Here's how the part is built. I have some questions about the finished solid (model axes, mm). Face numbers are marked on the shaded views. Give positions to 0.01 mm unless a question says otherwise; leave off trailing zeros. Loops run counter-clockwise (first coordinate to the right, second up) from the corner with the lowest first, then second, coordinate; pieces in that order, holes last. Notation, with made-up numbers: (-32.75, 53.5) - (14.25, 53.5) arc R23 ccw to (14.25, 66.5) - close; hole circle Ø7 at (40, 81). An arc over 180 degrees is marked (long way). Use a Markdown table: item, result.
from build123d import *

# Parameters (mm, degrees)
F0_R     = 1.1811
F0_R_2   = 1.5875
F1_DEPTH = 0.79375
F2_SIZE2 = 0.127
F2_SIZE  = 0.127


with BuildPart() as f1:
    # F0 (on Front) → F1 (new body, symmetric)
    with BuildSketch(Plane.XZ):
        with BuildLine():
            Line((5.280381, 3.991776), (-7.04344, 3.991776))
            ThreePointArc((-7.04344, 3.991776), (-3.637121, -4.925726), (5.280381, -1.519407))
            Line((5.280381, -1.519407), (5.280381, 3.991776))
        make_face()
        with Locations((-0.881529, -3.777536)):
            Circle(F0_R, mode=Mode.SUBTRACT)
        with Locations((-0.881529, 1.236185)):
            Circle(F0_R_2, mode=Mode.SUBTRACT)
    extrude(amount=F1_DEPTH, both=True)

    # F2
    f2_edges = [f1.edges().sort_by_distance(p)[0] for p in [
        (-2.062629, -0.79375, -3.777536),
    ]]
    chamfer(f2_edges, length=F2_SIZE, length2=F2_SIZE2)


solid = f1.part
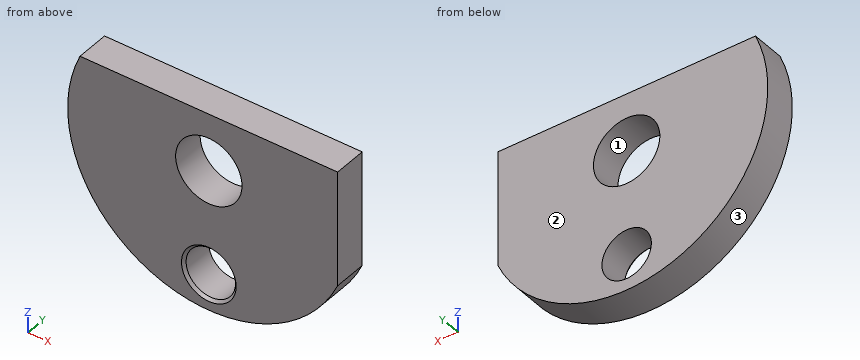
(1) Suppose I cut it at B-B on z = 2.5. Write out the boundary of the cut face in (x, y).
A:
| item | result |
|---|---|
| outline | (-7.51, -0.79) - (-1.84, -0.79) - (-1.84, 0.79) - (-7.51, 0.79) - close; (0.08, -0.79) - (5.28, -0.79) - (5.28, 0.79) - (0.08, 0.79) - close |
(2) Suppose I cut it at C-C on x = -1. Count the separate pieces of the cut face and the enclosed holes in it, plus the area to 3 significant figures.
A:
| item | result |
|---|---|
| separate pieces | 3 |
| enclosed holes | 0 |
| area | 6.31 mm2 |
(3) Suppose I cut it at A-A on z = 1.5. Write out the boundary of the cut face in (x, y).
A:
| item | result |
|---|---|
| outline | (-7.63, -0.79) - (-2.45, -0.79) - (-2.45, 0.79) - (-7.63, 0.79) - close; (0.68, -0.79) - (5.28, -0.79) - (5.28, 0.79) - (0.68, 0.79) - close |
(4) If I drill on line 1 (Z direction, x = -0.5, y = 0.5); line 2 (Z direction, x = -1, y = 0.4); line 3 (X direction, y = 0.3, z = -4), over which ranges is the centre line in solid material (lowest first)?
A:
| item | result |
|---|---|
| line 1 | -5.5 to -4.9, -2.66 to -0.3, 2.78 to 3.99 |
| line 2 | -5.51 to -4.95, -2.6 to -0.35, 2.82 to 3.99 |
| line 3 | -5.14 to -2.04, 0.28 to 3.38 |
(5) We'd pull the mould along X, two halves only. Please class the marked faces 1, 2 and 3: pulls with the +X half, pulls with the -X half, needs draft (parallel to the pull), parting line crosses it, or undercut.
A:
| item | result |
|---|---|
| face 1 | undercut |
| face 2 | needs draft |
| face 3 | parting line crosses it |
